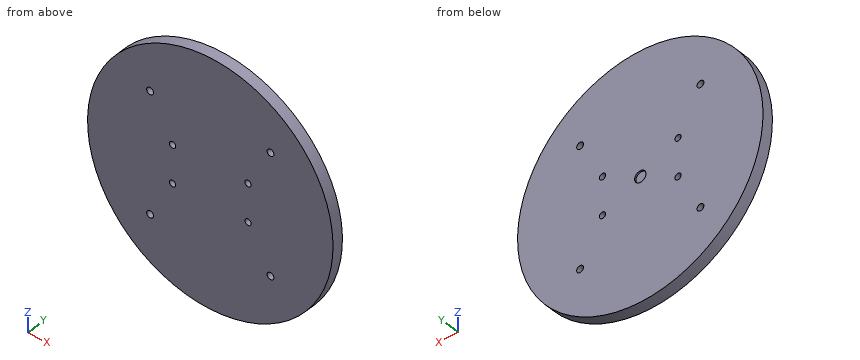
```python
from build123d import *

# Parameters (mm, degrees)
SKETCH1_R           = 82.55
SKETCH1_R_2         = 2.286
BOSS_EXTRUDE2_DEPTH = 7.62
SKETCH2_R           = 3.81
CUT_EXTRUDE1_DEPTH  = 1.016
SKETCH3_R           = 2.1
CUT_EXTRUDE2_DEPTH  = 54.356


with BuildPart() as part:
    # Sketch1 → Boss-Extrude2 (new body)
    with BuildSketch(Plane(origin=(0, 0, 0), x_dir=(1, 0, 0), z_dir=(0, 1, 0))):
        with Locations(Location((0, 0, 0), (0, 0, 90))):
            Circle(SKETCH1_R)
        with Locations(Location((40.49, 40.49, 0), (0, 0, 90))):
            Circle(SKETCH1_R_2, mode=Mode.SUBTRACT)
        with Locations(Location((40.49, -40.49, 0), (0, 0, 90))):
            Circle(SKETCH1_R_2, mode=Mode.SUBTRACT)
        with Locations(Location((-40.49, -40.49, 0), (0, 0, 90))):
            Circle(SKETCH1_R_2, mode=Mode.SUBTRACT)
        with Locations(Location((-40.49, 40.49, 0), (0, 0, 90))):
            Circle(SKETCH1_R_2, mode=Mode.SUBTRACT)
    extrude(amount=BOSS_EXTRUDE2_DEPTH)

    # Sketch2 → Cut-Extrude1 (cut)
    with BuildSketch(Plane(origin=(0, 7.62, 0), x_dir=(1, 0, 0), z_dir=(0, 1, 0))):
        with Locations(Location((0, 0, 0), (0, 0, 270))):
            Circle(SKETCH2_R)
    extrude(amount=-CUT_EXTRUDE1_DEPTH, mode=Mode.SUBTRACT)

    # Sketch3 → Cut-Extrude2 (cut)
    with BuildSketch(Plane.XZ):
        with Locations(Location((-25.4, 12.7, 0), (0, 0, 270))):
            Circle(SKETCH3_R)
        with Locations(Location((25.4, 12.7, 0), (0, 0, 270))):
            Circle(SKETCH3_R)
        with Locations(Location((25.4, -12.7, 0), (0, 0, 270))):
            Circle(SKETCH3_R)
        with Locations(Location((-25.4, -12.7, 0), (0, 0, 270))):
            Circle(SKETCH3_R)
    extrude(amount=-CUT_EXTRUDE2_DEPTH, mode=Mode.SUBTRACT)


solid = part.part
```
CAD build for the part. Positions are in the model's coordinates, mm. Round coordinates to 2 decimals unless told otherwise and drop trailing zeros. Loops run counter-clockwise (first coordinate to the right, second up) from the corner with the lowest first, then second, coordinate; pieces in that order, holes last. Notation, with made-up numbers: M 33.5,-35 L 86.5,-35 A19 ccw 86.5,-27 Z; hole C 84.25,25.5 d2. An arc over 180 degrees is marked long. Use a Markdown table: item, result. Add a question column.
(1) Cut at B-B (x = 25.4). Give the cut face in (y, z), and give its area (3 significant figures).
(2) Cut at D-D (z = -29.5). Give the cut face in (x, y), and give its area (3 significant figures).
(3) Cut at C-C (z = 12.7). Give the cut face in (x, y).
(4) Drill centre lines: line 1 (Z direction, x = 42.5, y = 2); line 2 (X direction, y = 7.1, z = 0); line 3 (X direction, y = 3.5, z = 40.49). Where is each one in solid material? Low to high.
(5) Flat gauge pins, fed straight in: pin 1 (1 mm diameter, centred on y = 1.5, z = 37, fed in from +X); pin 2 (6 mm diameter, centred on x = 0, z = 0, fed in from +Y); pin 3 (3 mm diameter, centred on x = 12.5, y = 4, fed in from -Z). Where does each tip first touch, or does it go through?
(6) Cut at A-A (y = 3.25). State how many separate pieces and enclosed holes the cut face has, and give its area (3 significant figures).
Geometry says:
| question | item | result |
|---|---|---|
| 1 | outline | M 0,-78.55 L 7.62,-78.55 L 7.62,-14.8 L 0,-14.8 Z; M 0,-10.6 L 7.62,-10.6 L 7.62,10.6 L 0,10.6 Z; M 0,14.8 L 7.62,14.8 L 7.62,78.55 L 0,78.55 Z |
| 1 | area | 1,130 mm² |
| 2 | outline | M -77.1,0 L 77.1,0 L 77.1,7.62 L -77.1,7.62 Z |
| 2 | area | 1,170 mm² |
| 3 | outline | M -81.57,0 L -27.5,0 L -27.5,7.62 L -81.57,7.62 Z; M -23.3,0 L 23.3,0 L 23.3,7.62 L -23.3,7.62 Z; M 27.5,0 L 81.57,0 L 81.57,7.62 L 27.5,7.62 Z |
| 4 | line 1 | z = -70.77 to -41.58, -39.4 to 39.4, 41.58 to 70.77 |
| 4 | line 2 | x = -82.55 to -3.81, 3.81 to 82.55 |
| 4 | line 3 | x = -71.94 to -42.78, -38.2 to 38.2, 42.78 to 71.94 |
| 5 | pin 1 | stops at x = 74.04 |
| 5 | pin 2 | stops at y = 6.6 |
| 5 | pin 3 | stops at z = -81.81 |
| 6 | separate pieces | 1 |
| 6 | enclosed holes | 8 |
| 6 | area | 21,300 mm² |
